from build123d import *

# Parameters (mm, degrees)
SKETCH2_R           = 1
BOSS_EXTRUDE1_DEPTH = 8.8
CUT_EXTRUDE1_DEPTH  = 1


with BuildPart() as part:
    # Sketch1 → Revolve1 (revolve)
    with BuildSketch(Plane(origin=(0, 0, 0), x_dir=(0, 0, -1), z_dir=(1, 0, 0))):
        Polygon((0, 0), (-1.9, 0), (-1, -0.9), (-1, -1.2), (0, -1.2), align=None)
    revolve(axis=Axis((0, 0.872326939, 0), (0, -1, 0)))

    # Sketch2 → Boss-Extrude1 (add)
    with BuildSketch(Plane.XZ.offset(1.2)):
        Circle(SKETCH2_R)
    extrude(amount=BOSS_EXTRUDE1_DEPTH)

    # Sketch3 → Cut-Extrude1 (cut)
    with BuildSketch(Plane(origin=(0, 0, 0), x_dir=(1, 0, 0), z_dir=(0, 1, 0))):
        with BuildLine():
            Line((-0.9, -0.2), (-0.4, -0.2))
            ThreePointArc((-0.4, -0.2), (-0.258578644, -0.258578644), (-0.2, -0.4))
            Line((-0.2, -0.4), (-0.2, -0.9))
            Line((-0.2, -0.9), (0.2, -0.9))
            Line((0.2, -0.9), (0.2, -0.4))
            ThreePointArc((0.2, -0.4), (0.258578644, -0.258578644), (0.4, -0.2))
            Line((0.4, -0.2), (0.9, -0.2))
            Line((0.9, -0.2), (0.9, 0.2))
            Line((0.9, 0.2), (0.4, 0.2))
            ThreePointArc((0.4, 0.2), (0.258578644, 0.258578644), (0.2, 0.4))
            Line((0.2, 0.4), (0.2, 0.9))
            Line((0.2, 0.9), (-0.2, 0.9))
            Line((-0.2, 0.9), (-0.2, 0.4))
            ThreePointArc((-0.2, 0.4), (-0.258578644, 0.258578644), (-0.4, 0.2))
            Line((-0.4, 0.2), (-0.9, 0.2))
            Line((-0.9, 0.2), (-0.9, -0.2))
        make_face()
    extrude(amount=-CUT_EXTRUDE1_DEPTH, mode=Mode.SUBTRACT)


solid = part.part
CAD build for the part. Positions are in the model's coordinates, mm. Coordinates: 2 decimals unless noted, no trailing zeros. Write each loop counter-clockwise with the first axis right and the second up, starting at its lowest first coordinate (ties: lowest second). Pieces come first, ordered by that corner, then holes. Notation, with made-up numbers: (32.5, 77) - (84.5, 77) arc R37 ccw to (84.5, 113) - close; hole circle Ø10 at (84, 12.25). An arc over 180 degrees is marked (long way). Use a Markdown table: item, result. Add a question column.
Item 1: Drill centre lines: L1, parallel to Y at x = -0.3, z = 0.15; L2, parallel to Z at x = -0.05, y = -1.75; L3, parallel to Z at x = -0.35, y = -0.5. Where is each one in solid material? Low to high. Write a range as from..to.
Item 2: Flat gauge pins, fed straight in: pin 1 (0.6 mm diameter, centred on x = 0.5, y = -0.5, fed in from +Z); pin 2 (1.5 mm diameter, centred on x = 1, y = -5, fed in from +Z); pin 3 (0.6 mm diameter, centred on y = -0.5, z = -0.5, fed in from +X). Where does each tip first touch, or does it go through?
Item 3: Mould opens along Z. For faces 1 (the face through (0, -10, 0)), 2 (the face through (0, -1, 0)) say: pulls with the +Z half, pulls with the -Z half, needs draft (parallel to the pull), parting line crosses it, or undercut.
Item 4: Band-saw the part on C-C, the plane y = -1.5. Give the cut face in (x, z).
Item 5: Band-saw the part on A-A, the plane x = 0. Give the cut face in (y, z), and give its area (3 significant figures).
Item 6: Band-saw the part on B-B, the plane z = 0. Give the cut face in (x, y), and give its area (3 significant figures).
Numbers:
| question | item | result |
|---|---|---|
| 1 | L1 | -10..-1 |
| 1 | L2 | -1..1 |
| 1 | L3 | -1.36..-0.21, 0.21..1.36 |
| 2 | pin 1 | z = 1.64 |
| 2 | pin 2 | z = 0.97 |
| 2 | pin 3 | x = 1.64 |
| 3 | face 1 | needs draft |
| 3 | face 2 | undercut |
| 4 | outline | circle Ø2 at (0, 0) |
| 5 | outline | (-10, -1) - (-0.9, -1) - (0, -1.9) - (0, -0.9) - (-1, -0.9) - (-1, 0.9) - (0, 0.9) - (0, 1.9) - (-0.9, 1) - (-10, 1) - close |
| 5 | area | 19.0 mm2 |
| 6 | outline | (-1.9, 0) - (-1, -0.9) - (-1, -10) - (1, -10) - (1, -0.9) - (1.9, 0) - (0.9, 0) - (0.9, -1) - (-0.9, -1) - (-0.9, 0) - close |
| 6 | area | 19.0 mm2 |
